For this review, take the finished solid that the model builds, in its own axes (mm). Face numbers are marked on the shaded views. A direction names the side the tool comes from. Coordinates: 2 decimals unless noted, no trailing zeros. Write each loop counter-clockwise with the first axis right and the second up, starting at its lowest first coordinate (ties: lowest second). Pieces come first, ordered by that corner, then holes. Notation, with made-up numbers: M 77,-10.5 L 131,-10.5 A6 cw 131,-3.5 Z; hole C -4.75,-23.5 d9. An arc over 180 degrees is marked long. One line per question, with ' | ' between items.
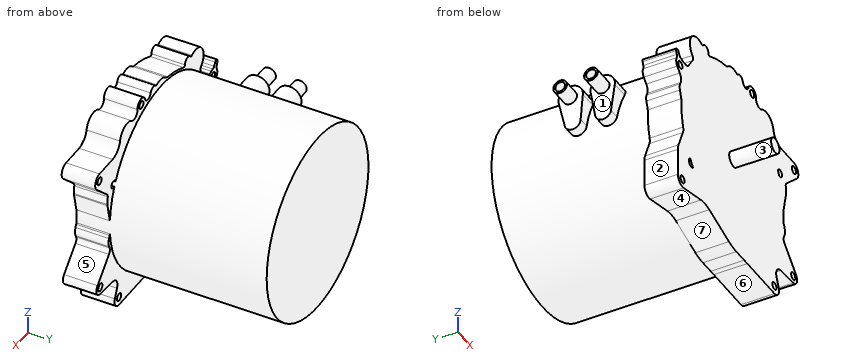
from build123d import *

# Parameters (mm, degrees)
SKETCH_R      = 10
PAD_DEPTH     = 55
SKETCH001_R   = 5
SKETCH001_R_2 = 5.752102
PAD001_DEPTH  = 44
SKETCH002_R   = 122
PAD002_DEPTH  = 250
PAD003_DEPTH  = 137
SKETCH004_R   = 9.029167
SKETCH004_R_2 = 6.410546
PAD004_DEPTH  = 28
SKETCH005_R   = 9.029167
SKETCH005_R_2 = 6.410546
PAD005_DEPTH  = 24


with BuildPart() as part:
    # Sketch → Pad (new body)
    with BuildSketch(Plane.XZ):
        Circle(SKETCH_R)
    extrude(amount=PAD_DEPTH)

    # Sketch001 → Pad001 (join)
    with BuildSketch(Plane.XZ):
        with BuildLine():
            ThreePointArc((96.175862, 107.050758), (85.01162, 120.214268), (67.94679, 117.623927))
            ThreePointArc((54.367316, 124.71944), (58.880143, 116.814107), (67.94679, 117.623927))
            ThreePointArc((54.367316, 124.71944), (46.670454, 134.337495), (36.21786, 127.81891))
            ThreePointArc((22.758705, 127.681071), (29.539283, 122.770138), (36.21786, 127.81891))
            ThreePointArc((22.758705, 127.681071), (17.601424, 132.416088), (10.911961, 130.349928))
            ThreePointArc((8.144721, 129.75708), (9.62161, 129.618152), (10.911961, 130.349928))
            ThreePointArc((8.144721, 129.75708), (-3.17481, 131.027317), (-13.371145, 125.949913))
            ThreePointArc((-18.099593, 123.682678), (-15.562998, 124.456805), (-13.371145, 125.949913))
            ThreePointArc((-18.099593, 123.682678), (-37.745711, 119.164849), (-56.410125, 111.547738))
            ThreePointArc((-59.467861, 113.415794), (-58.459377, 111.629973), (-56.410125, 111.547738))
            ThreePointArc((-59.467861, 113.415794), (-64.373735, 119.916678), (-72.004271, 117.069923))
            ThreePointArc((-76.03682, 116.00781), (-73.814492, 115.756539), (-72.004271, 117.069923))
            ThreePointArc((-76.03682, 116.00781), (-100.534649, 110.217356), (-98.248389, 85.148531))
            ThreePointArc((-97.764943, 77.891051), (-96.600774, 81.613442), (-98.248389, 85.148531))
            ThreePointArc((-97.764943, 77.891051), (-102.377192, 71.721061), (-106.600626, 65.278684))
            ThreePointArc((-114.445294, 60.883833), (-109.949364, 62.057409), (-106.600626, 65.278684))
            Line((-118.727486, 60.883833), (-114.445294, 60.883833))
            ThreePointArc((-122.640758, 61.745456), (-120.730989, 61.101788), (-118.727486, 60.883833))
            ThreePointArc((-122.640758, 61.745456), (-124.406768, 62.380022), (-126.256912, 62.693763))
            ThreePointArc((-129.326019, 64.601052), (-128.023095, 63.274682), (-126.256912, 62.693763))
            Line((-129.326019, 64.601052), (-131.922169, 68.949759))
            ThreePointArc((-131.922169, 68.949759), (-135.945808, 70.073625), (-137.270814, 66.111667))
            Line((-135.647932, 61.659144), (-137.270814, 66.111667))
            ThreePointArc((-135.958333, 56.645211), (-135.280116, 59.119799), (-135.647932, 61.659144))
            ThreePointArc((-135.958333, 56.645211), (-136.967186, 50.815076), (-134.488163, 45.442673))
            Line((-128.394518, 39.452321), (-134.488163, 45.442673))
            ThreePointArc((-126.12643, 27.585779), (-125.408538, 33.873016), (-128.394518, 39.452321))
            Line((-127.60596, 24.238917), (-126.12643, 27.585779))
            ThreePointArc((-127.60596, 24.238917), (-128.700482, 19.721553), (-128.147111, 15.106542))
            Line((-124.916008, 4.581578), (-128.147111, 15.106542))
            ThreePointArc((-124.916008, 4.581578), (-124.14364, -14.606734), (-120.441181, -33.45029))
            ThreePointArc((-120.957831, -41.567166), (-120.014396, -37.552337), (-120.441181, -33.45029))
            Line((-131.420927, -66.450927), (-120.957831, -41.567166))
            ThreePointArc((-131.420927, -66.450927), (-132.541496, -70.092422), (-132.92, -73.883583))
            Line((-132.92, -73.883583), (-132.92, -110.12))
            ThreePointArc((-132.92, -110.12), (-128.693171, -118.787419), (-119.261062, -120.793802))
            Line((-77.676912, -110.434825), (-119.261062, -120.793802))
            ThreePointArc((-57.595038, -111.058963), (-67.59276, -109.356427), (-77.676912, -110.434825))
            Line((-57.595038, -111.058963), (-10.608757, -125.917415))
            ThreePointArc((-10.608757, -125.917415), (-1.840442, -127.933804), (7.137416, -128.523075))
            Line((7.137416, -128.523075), (26.044697, -128.245047))
            ThreePointArc((33.531981, -128.19), (29.788238, -128.203762), (26.044697, -128.245047))
            Line((33.531981, -128.19), (98.52, -128.19))
            ThreePointArc((98.52, -128.19), (107.693886, -123.259581), (108.643935, -112.888147))
            Line((108.643935, -112.888147), (103.568399, -100.943433))
            ThreePointArc((113.34084, -84.800022), (104.323208, -90.37077), (103.568399, -100.943433))
            Line((113.34084, -84.800022), (144.283252, -82.30988))
            ThreePointArc((144.283252, -82.30988), (152.354382, -76.160143), (150.121204, -66.261894))
            Line((150.121204, -66.261894), (122.754449, -39.291647))
            ThreePointArc((121.283431, -30.889473), (120.674662, -35.32591), (122.754449, -39.291647))
            Line((122.493763, -28.358461), (121.283431, -30.889473))
            ThreePointArc((122.493763, -28.358461), (123.902721, -22.337711), (122.659289, -16.280611))
            Line((121.143318, -12.873569), (122.659289, -16.280611))
            ThreePointArc((119.540487, 3.52367), (119.013733, -4.804778), (121.143318, -12.873569))
            Line((126.394372, 33.640226), (119.540487, 3.52367))
            ThreePointArc((126.394372, 33.640226), (126.522404, 34.506324), (126.516063, 35.38181))
            Line((125.62119, 45.978723), (126.516063, 35.38181))
            ThreePointArc((127.371051, 50.552529), (125.973127, 48.465714), (125.62119, 45.978723))
            Line((152.523328, 74.255672), (127.371051, 50.552529))
            ThreePointArc((152.523328, 74.255672), (155.085641, 85.790421), (145.31, 92.427644))
            Line((113.958558, 92.427644), (145.31, 92.427644))
            ThreePointArc((96.175862, 107.050758), (102.447045, 96.552903), (113.958558, 92.427644))
        make_face()
        with Locations((145.31, 81.91)):
            Circle(SKETCH001_R, mode=Mode.SUBTRACT)
        with Locations((45.11, 125.2)):
            Circle(SKETCH001_R, mode=Mode.SUBTRACT)
        with Locations((143.53, -72.95)):
            Circle(SKETCH001_R, mode=Mode.SUBTRACT)
        with Locations((98.52, -117.19)):
            Circle(SKETCH001_R, mode=Mode.SUBTRACT)
        with Locations((-121.92, -110.12)):
            Circle(SKETCH001_R, mode=Mode.SUBTRACT)
        with Locations((-127.1, 52.11)):
            Circle(SKETCH001_R, mode=Mode.SUBTRACT)
        with Locations((111.87, 54.67)):
            Circle(SKETCH001_R, mode=Mode.SUBTRACT)
        with Locations((-100.79, -72.38)):
            Circle(SKETCH001_R_2, mode=Mode.SUBTRACT)
    extrude(amount=-PAD001_DEPTH)

    # Sketch002 → Pad002 (join)
    with BuildSketch(Plane.XZ):
        with Locations((-1.164187, -0.6689)):
            Circle(SKETCH002_R)
    extrude(amount=-PAD002_DEPTH)

    # Sketch003 → Pad003 (join)
    with BuildSketch(Plane(origin=(0, 0, 0), x_dir=(0, 1, -0.000994), z_dir=(1, 0, 0))):
        with BuildLine():
            ThreePointArc((154.118951, 45.729048), (139.583053, 65.163428), (122.55534, 47.870527))
            Line((125.500082, 12.556877), (122.55534, 47.870527))
            ThreePointArc((125.500082, 12.556877), (134.874857, 2.158872), (146.249936, 10.320521))
            Line((146.249936, 10.320521), (154.118951, 45.729048))
        make_face()
        with BuildLine():
            ThreePointArc((112.284143, 46.589719), (96.718502, 65.207545), (80.65021, 47.021765))
            Line((85.598581, 11.164033), (80.65021, 47.021765))
            ThreePointArc((85.598581, 11.164033), (95.856629, 2.100452), (106.358344, 10.880544))
            Line((106.358344, 10.880544), (112.284143, 46.589719))
        make_face()
    extrude(amount=-PAD003_DEPTH)

    # Sketch004 (on Face91 of Pad003) → Pad004 (join)
    with BuildSketch(Plane(origin=(-137, 0, 0), x_dir=(0, 0, -1), z_dir=(-1, 0, 0))):
        with Locations((-48.752483, -96.561478)):
            Circle(SKETCH004_R)
        with Locations((-48.752483, -96.561478)):
            Circle(SKETCH004_R_2, mode=Mode.SUBTRACT)
    extrude(amount=PAD004_DEPTH)

    # Sketch005 (on Face90 of Pad004) → Pad005 (join)
    with BuildSketch(Plane(origin=(-137, 0, 0), x_dir=(0, 0, -1), z_dir=(-1, 0, 0))):
        with Locations((-48.752483, -139.271042)):
            Circle(SKETCH005_R)
        with Locations((-48.752483, -139.271042)):
            Circle(SKETCH005_R_2, mode=Mode.SUBTRACT)
    extrude(amount=PAD005_DEPTH)


solid = part.part
1. Take a section at B-B on y = 229. State the section outline as (x, z) points, plus the area to 3 significant figures.
Computed values:
outline: C -1.16,-0.67 d244 | area: 46,800 mm2
2. Clearance check with flat-ended pins moving along their axes: P1, Ø1.3, axis at x = -117, y = 19, coming from the +Z side; P2, Ø6, axis at x = 58.5, z = 81, coming from the -Y side; P3, Ø2, axis at x = -28, y = 126, coming from the -Z side. State where each tip first meets the part, or that it passes through.
Computed values:
P1: stops at z = 60.88 | P2: stops at y = 0 | P3: stops at z = -119.9
3. Take a section at A-A on x = 45. State the section outline as (y, z) points.
Computed values:
outline: M 0,-128.19 L 44,-128.19 L 44,-113.6 L 250,-113.6 L 250,112.26 L 44,112.26 L 44,120.2 L 0,120.2 Z; M 0,130.2 L 44,130.2 L 44,134.47 L 0,134.47 Z
4. Machinability: for the marked faces 1, 2, 3 and 4, which of the approach directions +Z, -Z, +X, -X, +Y, -Y give a long, thin tool a straight path to every point of the face, cutting with its end or side? Answer none if there is none.
Computed values:
face 1: -X | face 2: -Z, -X, +Y, -Y | face 3: -Y | face 4: -Z, +Y, -Y
5. Draft analysis for pull direction X (two halves, no side actions). For the marked faces 5, 6 and 7, state which applies: pulls with the +X half, pulls with the -X half, needs draft (parallel to the pull), parting line crosses it, or undercut.
Computed values:
face 5: pulls with the +X half | face 6: needs draft | face 7: undercut
6. For line 1 along Y through (x, z) = (-94.5, -51.5); line 2 along Z through (x, y) = (-13, 144); line 3 along Z through (x, y) = (98.52, 20.5), list the stretches that pass through material, from the lowest coordinate up.
Computed values:
line 1: y = 0 to 250 | line 2: z = -122.09 to 120.76 | line 3: z = -128.19 to -122.19, -112.19 to 101.06
